Geometry: final body of the model. Coordinates: model frame, mm. Face numbers are marked on the shaded views. Give positions to 0.01 mm unless a question says otherwise; leave off trailing zeros. Write each loop counter-clockwise with the first axis right and the second up, starting at its lowest first coordinate (ties: lowest second). Pieces come first, ordered by that corner, then holes.
Q1. Section B-B (x = 0). Return the cut outline in (y, z).
Q2. Line query: line 1 (Y direction, x = -17, z = -37.5); line 2 (X direction, y = 16, z = -36.5); line 3 (Y direction, x = 0, z = -14). Output: solid intervals per line, ascending.
Q3. Pin query (flat end, axial travel): pin 1 Ø2.5 at (x, y) = (-16.66, -16.74) entering from -Z. Return the tip coordinate at first contact, or that it passes through.
Q4. Section A-A (y = 0). Return the cut outline in (x, z).
Q5. Section C-C (z = -3.5). Return the cut outline in (x, y), plus the area to 3 significant figures.
Q6. Mould query, pull axis Y, two halves, no side actions, for the marked faces 1, 2, 3 and 4. Classes: +Y half, -Y half, draft (parallel to the pull), parting line (faces both ways), or undercut.
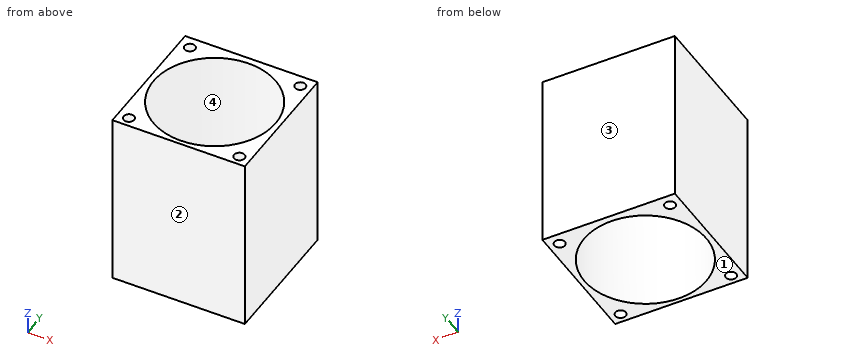
from build123d import *

# Parameters (mm, degrees)
F0_W   = 40
F0_H   = 40
F0_R   = 1.6
F0_R_2 = 18.4155


with BuildPart() as f2:
    # F2: sweep along a path in F1
    with BuildLine(Plane.YZ) as f2_path:
        Line((0, 0), (0, -54))
    # F0 (on Top) → F2 (sweep)
    with BuildSketch(Plane.XY):
        with Locations((-0.088266, 0.357345)):
            Rectangle(F0_W, F0_H)
        with Locations((-16.664036, -16.74399)):
            Circle(F0_R, mode=Mode.SUBTRACT)
        with Locations((16.664036, -16.74399)):
            Circle(F0_R, mode=Mode.SUBTRACT)
        Circle(F0_R_2, mode=Mode.SUBTRACT)
        with Locations((-16.664036, 16.74399)):
            Circle(F0_R, mode=Mode.SUBTRACT)
        with Locations((16.664036, 16.74399)):
            Circle(F0_R, mode=Mode.SUBTRACT)
    sweep(path=f2_path.line)


solid = f2.part
Computed:
1. outline: (-19.64, -54) - (-18.42, -54) - (-18.42, 0) - (-19.64, 0) - close; (18.42, -54) - (20.36, -54) - (20.36, 0) - (18.42, 0) - close
2. line 1: y = -19.64 to -18.31, -15.18 to -7.08, 7.08 to 15.18, 18.31 to 20.36
2. line 2: x = -20.09 to -18.08, -15.25 to -9.12, 9.12 to 15.25, 18.08 to 19.91
2. line 3: y = -19.64 to -18.42, 18.42 to 20.36
3. pin 1: passes through
4. outline: (-20.09, -54) - (-18.42, -54) - (-18.42, 0) - (-20.09, 0) - close; (18.42, -54) - (19.91, -54) - (19.91, 0) - (18.42, 0) - close
5. outline: (-20.09, -19.64) - (19.91, -19.64) - (19.91, 20.36) - (-20.09, 20.36) - close; hole circle Ø36.83 at (0, 0); hole circle Ø3.2 at (-16.66, -16.74); hole circle Ø3.2 at (-16.66, 16.74); hole circle Ø3.2 at (16.66, -16.74); hole circle Ø3.2 at (16.66, 16.74)
5. area: 502 mm2
6. face 1: draft
6. face 2: -Y half
6. face 3: +Y half
6. face 4: undercut
